Here's the drawing with two shaded views (mm, measured from the low corner). I have some questions. A direction names the side the tool comes from. Round coordinates to 2 decimals unless told otherwise and drop trailing zeros. Order: outer loops, then holes, each group sorted by start corner. A loop starts at its lowest first (then second) coordinate and runs counter-clockwise, first axis right, second up. Notation, with made-up numbers: (-24, 69) - (29, 69) arc R20 ccw to (29, 74) - close; hole circle Ø9 at (25.5, 28). An arc over 180 degrees is marked (long way). One line per item, written item: value.
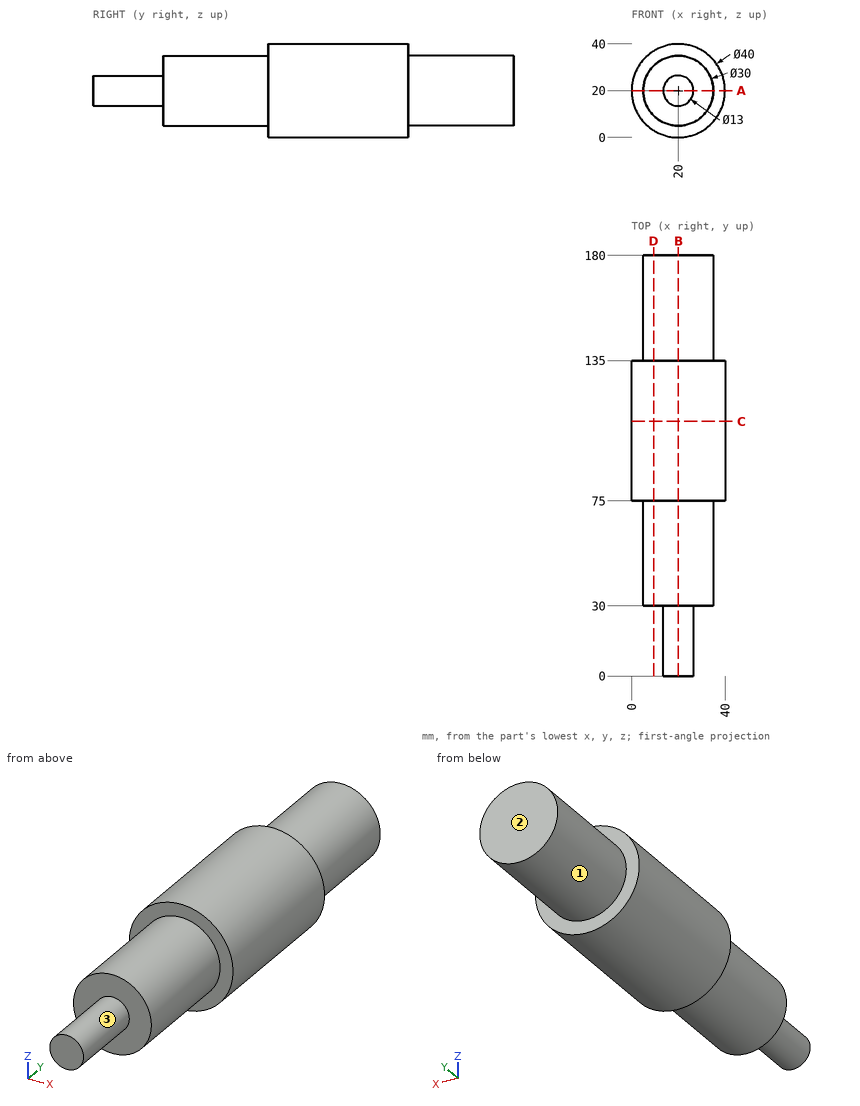
Q1. Which directions (+Z, -Z, +X, -X, +Y, -Y) give clear straight access to the entire face, cutting with the end or side of a thin tool? Please do the marked faces 1, 2 and 3.
Results list:
face 1: +Y
face 2: +Z, -Z, +X, -X, +Y
face 3: -Y
Q2. If we section it at D-D, the plane x = 9.5: Please give me the cut outline in (y, z).
Results list:
outline: (30, 9.29) - (75, 9.29) - (75, 2.98) - (135, 2.98) - (135, 9.29) - (180, 9.29) - (180, 30.71) - (135, 30.71) - (135, 37.02) - (75, 37.02) - (75, 30.71) - (30, 30.71) - close
Q3. If we section it at B-B, the plane x = 20: Please give me the cut outline in (y, z), then the cut area to 3 significant figures.
Results list:
outline: (0, 13.5) - (30, 13.5) - (30, 5) - (75, 5) - (75, 0) - (135, 0) - (135, 5) - (180, 5) - (180, 35) - (135, 35) - (135, 40) - (75, 40) - (75, 35) - (30, 35) - (30, 26.5) - (0, 26.5) - close
area: 5,490 mm²
Q4. If I drill on line 1 along Y through (x, z) = (26, 30); line 2 along Y through (x, z) = (22, 38); line 3 along Z through (x, y) = (19, 129.5), over which ranges is the centre line in solid material (lowest first)?
Results list:
line 1: 30 to 180
line 2: 75 to 135
line 3: 0.03 to 39.97
Q5. Will these pins go through, and if not, where does the flat tip stop? pin 1 (4 mm diameter, centred on x = 12, z = 21, fed in from -Y); pin 2 (6 mm diameter, centred on x = 22, z = 32, fed in from -Y); pin 3 (1 mm diameter, centred on y = 47, z = 6, fed in from +X); pin 4 (5 mm diameter, centred on y = 18, z = 25, fed in from -X).
Results list:
pin 1: y = 0
pin 2: y = 30
pin 3: x = 26.54
pin 4: x = 14
Q6. If we section it at C-C, the plane y = 109: Please give me the cut outline in (x, z), then the cut area to 3 significant figures.
Results list:
outline: circle Ø40 at (20, 20)
area: 1,260 mm²
Q7. If we section it at A-A, the plane z = 20: Please give me the cut outline in (x, y), then the cut area to 3 significant figures.
Results list:
outline: (0, 75) - (5, 75) - (5, 30) - (13.5, 30) - (13.5, 0) - (26.5, 0) - (26.5, 30) - (35, 30) - (35, 75) - (40, 75) - (40, 135) - (35, 135) - (35, 180) - (5, 180) - (5, 135) - (0, 135) - close
area: 5,490 mm²
